from build123d import *

# Parameters (mm, degrees)
SKETCH1_R           = 54
BOSS_EXTRUDE1_DEPTH = 10
CUT_EXTRUDE1_START  = -10
CUT_EXTRUDE1_DEPTH  = 10
CIRPATTERN1_COUNT   = 16
CUT_EXTRUDE2_START  = -10
CUT_EXTRUDE2_DEPTH  = 10
SKETCH5_R           = 4.25
CUT_EXTRUDE3_DEPTH  = 10


with BuildPart() as part:
    # Sketch1 → Boss-Extrude1 (new body)
    with BuildSketch(Plane.XY):
        Circle(SKETCH1_R)
    extrude(amount=BOSS_EXTRUDE1_DEPTH)

    # Sketch2 → Cut-Extrude1 (cut)
    with BuildSketch(Plane.XY.offset(10).offset(CUT_EXTRUDE1_START)):
        with BuildLine():
            ThreePointArc((-2.226451575, 40.937500136), (-0.390558879, 44.240929479), (0, 48))
            ThreePointArc((0, 48), (0.916562017, 51.223157404), (2.90289612, 53.921917567))
            ThreePointArc((2.90289612, 53.921917567), (-5.3015625, 53.739123877), (-13.383578744, 52.315196836))
            ThreePointArc((-13.383578744, 52.315196836), (-10.908183383, 50.056602718), (-9.379467454, 47.07468099))
            ThreePointArc((-9.379467454, 47.07468099), (-8.261894241, 43.464393254), (-5.815884428, 40.583389365))
            ThreePointArc((-5.815884428, 40.583389365), (-4.025064063, 40.79993705), (-2.226451575, 40.937500136))
        make_face()
    cut_extrude1 = extrude(amount=CUT_EXTRUDE1_DEPTH, mode=Mode.SUBTRACT)

    # CirPattern1: Cut-Extrude1 ×16 about axis
    cirpattern1_axis = Axis((0, 0, 0), (0, 0, 1))
    for i in range(1, CIRPATTERN1_COUNT):
        add(cut_extrude1.rotate(cirpattern1_axis, i * 360 / CIRPATTERN1_COUNT), mode=Mode.SUBTRACT)

    # Sketch4 → Cut-Extrude2 (cut)
    with BuildSketch(Plane.XY.offset(10).offset(CUT_EXTRUDE2_START)):
        with BuildLine():
            ThreePointArc((-31.696062253, 26.003762067), (-19.456690994, 36.087022315), (-4.306352435, 40.771207153))
            Line((-4.306352435, 40.771207153), (-5.672057942, 53.701282654))
            ThreePointArc((-5.672057942, 53.701282654), (-41.865929649, 34.106362085), (-53.739123877, -5.3015625))
            Line((-53.739123877, -5.3015625), (-40.79993705, -4.025064063))
            ThreePointArc((-40.79993705, -4.025064063), (-39.234552099, 11.894785646), (-31.696062253, 26.003762067))
        make_face()
        with BuildLine():
            ThreePointArc((-4.306352435, 40.771207153), (40.771207153, 4.306352435), (4.306352435, -40.771207153))
            Line((4.306352435, -40.771207153), (5.672057942, -53.701282654))
            ThreePointArc((5.672057942, -53.701282654), (53.701282654, 5.672057942), (-5.672057942, 53.701282654))
            Line((-5.672057942, 53.701282654), (-4.306352435, 40.771207153))
        make_face()
    extrude(amount=CUT_EXTRUDE2_DEPTH, mode=Mode.SUBTRACT)

    # Sketch5 → Cut-Extrude3 (cut)
    with BuildSketch(Plane.XY.offset(10)):
        Circle(SKETCH5_R)
    extrude(amount=-CUT_EXTRUDE3_DEPTH, mode=Mode.SUBTRACT)


solid = part.part
Can you work these out from the model? Positions are in its coordinate system, mm. A direction names the side the tool comes from. Give positions to 0.01 mm unless a question says otherwise; leave off trailing zeros. Write each loop counter-clockwise with the first axis right and the second up, starting at its lowest first coordinate (ties: lowest second). Pieces come first, ordered by that corner, then holes. Notation, with made-up numbers: (-5.5, 4.5) -> (29.5, 4.5) arc R32 ccw to (29.5, 33.5) -> close; hole circle Ø5 at (64, 14). An arc over 180 degrees is marked (long way). Answer as a JSON object with one key per item and string values. Group by question number.
Item 1: Suppose I cut it at B-B (x = -22). Please give me the cut outline in (y, z).
Item 2: I'm going to push flat-ended pins straight in: P1, Ø6, axis at y = -41.5, z = 2.5, coming from the -X side; P2, Ø5, axis at y = -24, z = 2.5, coming from the -X side. Where does each tip first touch, or does it pass through?
Item 3: For faces 1 (the face through (-24.9, -36.6, 4.9)), 2 (the face through (-11.87, -39.24, 4.93)), 3 (the face through (-37.03, -24.31, 4.93)), which set-ups out of +Z, -Z, +X, -X, +Y, -Y let a thin tool reach every point of the face, with its end or its side?
Item 4: Suppose I cut it at C-C (y = 16). Please give me the cut outline in (x, z).
Item 5: Please list where these lines run through material, in increasing order: line 1 (Y direction, x = -41.5, z = 4.5) (3 decimals); line 2 (Y direction, x = 3.5, z = 6.25); line 3 (Y direction, x = -5.5, z = 7.5). Write a range as [from, to].
Item 6: We'd pull the mould along X, two halves only. Please class faces 4 (the face through (-36.824, -35.557, 4.93)), 5 (the face through (-51.682, -15.652, 4.93)), 6 (the face through (-30.96, -31.535, 4.93)), 7 (the face through (-0.896, -51.181, 4.93)): +X half, -X half, draft (parallel to the pull), parting line (faces both ways), or undercut.
Item 7: Suppose I cut it at A-A (y = 0). Please give me the cut outline in (x, z), plus the area to 3 significant figures.
Findings:
{
 "1": {"outline": "(-48.08, 0) -> (34.6, 0) -> (34.6, 10) -> (-48.08, 10) -> close"},
 "2": {"P1": "stops at x = -27.77", "P2": "stops at x = -39.58"},
 "3": {"face 1": "+Z, -Z", "face 2": "+Z, -Z, -Y", "face 3": "+Z, -Z, -X"},
 "4": {"outline": "(-37.75, 0) -> (37.75, 0) -> (37.75, 10) -> (-37.75, 10) -> close"},
 "5": {"line 1": "y = [-34.551, -28.363], [-17.392, -6.825]", "line 2": "y = [-40.85, -2.41], [2.41, 40.85]", "line 3": "y = [-53.72, 40.63]"},
 "6": {"face 4": "undercut", "face 5": "-X half", "face 6": "undercut", "face 7": "+X half"},
 "7": {"outline": "(-41, 0) -> (-4.25, 0) -> (-4.25, 10) -> (-41, 10) -> close; (4.25, 0) -> (41, 0) -> (41, 10) -> (4.25, 10) -> close", "area": "735 mm²"}
}
